```python
from build123d import *

# Parameters (mm, degrees)
BOSS_EXTRUDE1_DEPTH = 60
SKETCH2_R           = 25
BOSS_EXTRUDE2_DEPTH = 16
BOSS_EXTRUDE4_DEPTH = 17
BOSS_EXTRUDE5_DEPTH = 38
SKETCH4_W           = 30
SKETCH4_H           = 23
CUT_EXTRUDE1_DEPTH  = 110


with BuildPart() as part:
    # Sketch1 → Boss-Extrude1 (new body)
    with BuildSketch(Plane.XY):
        Polygon((-55.432527154, -19.042703446), (-55.432527154, -27.042703446), (34.567472846, -27.042703446), (34.567472846, -19.042703446), (14.567472846, 4.957296554), (-35.432527154, 4.957296554), align=None)
    extrude(amount=BOSS_EXTRUDE1_DEPTH)

    # Sketch2 → Boss-Extrude2 (add)
    with BuildSketch(Plane(origin=(0, 4.957296554, 0), x_dir=(1, 0, 0), z_dir=(0, 1, 0))):
        with Locations(Location((-10.432527154, -30, 0), (0, 0, 180))):
            Circle(SKETCH2_R)
    extrude(amount=BOSS_EXTRUDE2_DEPTH)

    # Sketch3 → Boss-Extrude4 (add)
    with BuildSketch(Plane(origin=(0, 20.957296554, 0), x_dir=(1, 0, 0), z_dir=(0, 1, 0))):
        Polygon((1.567472846, -20), (-10.432527154, -20), (-22.432527154, -20), (-22.432527154, -40), (-10.432527154, -40), (1.567472846, -40), align=None)
    extrude(amount=BOSS_EXTRUDE4_DEPTH)

    # Sketch3_4 → Boss-Extrude5 (add)
    with BuildSketch(Plane(origin=(0, 20.957296554, 0), x_dir=(1, 0, 0), z_dir=(0, 1, 0))):
        with BuildLine():
            Line((-22.432527154, -40), (-22.432527154, -20))
            Line((-22.432527154, -20), (-33.345405628, -20))
            ThreePointArc((-33.345405628, -20), (-35.432527154, -30), (-33.345405628, -40))
            Line((-33.345405628, -40), (-22.432527154, -40))
        make_face()
        with BuildLine():
            Line((12.480351321, -20), (1.567472846, -20))
            Line((1.567472846, -20), (1.567472846, -40))
            Line((1.567472846, -40), (12.480351321, -40))
            ThreePointArc((12.480351321, -40), (14.04013067, -35.107741092), (14.567472846, -30))
            ThreePointArc((14.567472846, -30), (14.04013067, -24.892258908), (12.480351321, -20))
        make_face()
    extrude(amount=BOSS_EXTRUDE5_DEPTH)

    # Sketch4 → Cut-Extrude1 (cut)
    with BuildSketch(Plane(origin=(34.567472846, 0, 0), x_dir=(0, 0, -1), z_dir=(1, 0, 0))):
        with Locations((-30, -15.542703446)):
            Rectangle(SKETCH4_W, SKETCH4_H)
    extrude(amount=-CUT_EXTRUDE1_DEPTH, mode=Mode.SUBTRACT)


solid = part.part
```
Source: CAD feature listing. Evaluate the final solid. Frame: model axes, mm. A direction names the side the tool comes from. Coordinates: 2 decimals unless noted, no trailing zeros. Write each loop counter-clockwise with the first axis right and the second up, starting at its lowest first coordinate (ties: lowest second). Pieces come first, ordered by that corner, then holes. Notation, with made-up numbers: (19.25, 59.25) -> (61.25, 59.25) arc R16 ccw to (61.25, 79.25) -> close; hole circle Ø2 at (-11, -29.5). An arc over 180 degrees is marked (long way). Return JSON: item names as keys, results as strings. Group by question number.
1) Ray query, line 1 along X through (y, z) = (38.5, 30); line 2 along Z through (x, y) = (-7, -17.5); line 3 along Y through (x, z) = (-31.5, 37). Return the intervals inside material, ascending.
2) Section query C-C, the plane x = -1.5. Return loops of the section in (y, z), plus the area to 3 significant figures.
3) Set-up query: faces 1 (the face through (-10, -16, 45)), 2 (the face through (-12, 4.957, 56)), 3 (the face through (-22.433, 48, 30)). Return all of +Z, -Z, +X, -X, +Y, -Y with unobstructed straight access to the full face (end or side cutting, diameter ignored); none if empty.
4) Section query D-D, the plane y = 35.5. Return loops of the section in (x, z).
5) Contact query for flat-ended pins moving along their axis: P1, Ø22, axis at y = 47.5, z = 30, coming from the -X side; P2, Ø12, axis at y = 46.5, z = 28.5, coming from the +X side; P3, Ø6, axis at x = -26, z = 34.5, coming from the -Y side; P4, Ø2, axis at x = 17, y = 6.5, coming from the +Z side. Output: stop coordinate, or through.
6) Section query A-A, the plane y = -11. Return loops of the section in (x, z).
7) Section query B-B, the plane z = 34. Return loops of the section in (x, y).
8) Mould query, pull axis X, two halves, no side actions, for faces 4 (the face through (-55.433, -23, 52)), 5 (the face through (-11, 37.957, 30)), 6 (the face through (20.263, -1.877, 29.58)). Classes: +X half, -X half, draft (parallel to the pull), parting line (faces both ways), or undercut.
From the geometry:
{
 "1": {"line 1": "-35.43 to -22.43, 1.57 to 14.57", "line 2": "0 to 15, 45 to 60", "line 3": "-4.04 to 58.96"},
 "2": {"outline": "(-27.04, 0) -> (4.96, 0) -> (4.96, 6.65) -> (20.96, 6.65) -> (20.96, 20) -> (37.96, 20) -> (37.96, 40) -> (20.96, 40) -> (20.96, 53.35) -> (4.96, 53.35) -> (4.96, 60) -> (-27.04, 60) -> (-27.04, 45) -> (-4.04, 45) -> (-4.04, 15) -> (-27.04, 15) -> close", "area": "2,320 mm²"},
 "3": {"face 1": "+X, -X, -Y", "face 2": "+Z, +Y", "face 3": "+Z, -Z, +Y"},
 "4": {"outline": "(-33.35, 20) -> (12.48, 20) arc R25 ccw to (12.48, 40) -> (-33.35, 40) arc R25 ccw to start"},
 "5": {"P1": "x = -35.43", "P2": "x = 14.57", "P3": "y = -4.04", "P4": "through"},
 "6": {"outline": "(-48.73, 0) -> (27.87, 0) -> (27.87, 15) -> (-48.73, 15) -> close; (-48.73, 45) -> (27.87, 45) -> (27.87, 60) -> (-48.73, 60) -> close"},
 "7": {"outline": "(-42.93, -4.04) -> (22.07, -4.04) -> (14.57, 4.96) -> (14.25, 4.96) -> (14.25, 58.96) -> (1.57, 58.96) -> (1.57, 37.96) -> (-22.43, 37.96) -> (-22.43, 58.96) -> (-35.11, 58.96) -> (-35.11, 4.96) -> (-35.43, 4.96) -> close"},
 "8": {"face 4": "-X half", "face 5": "undercut", "face 6": "+X half"}
}
